```python
from build123d import *

# Parameters (mm, degrees)
F0_R     = 20
F0_R_2   = 10
F1_DEPTH = 28
F2_DEPTH = 40
F3_DEPTH = 12


with BuildPart() as f1:
    # F0 (on Front) → F1 (new body)
    with BuildSketch(Plane.XZ):
        Circle(F0_R)
        Circle(F0_R_2, mode=Mode.SUBTRACT)
    extrude(amount=F1_DEPTH)



with BuildPart() as f2:
    # F0 (on Front) → F2 (new body)
    with BuildSketch(Plane.XZ):
        Polygon((40, -40), (0, -40), (-40, -40), (-40, -70), (-20, -70), (-20, -55), (20, -55), (20, -70), (40, -70), align=None)
    extrude(amount=F2_DEPTH)


with BuildPart() as f1_1:
    add(f1.part)

    add(f2.part)  # F3 merges F2
    # F0 (on Front) → F3 (join)
    with BuildSketch(Plane.XZ):
        with BuildLine():
            ThreePointArc((0, -40), (28.2842712475, -28.2842712475), (40, 0))
            ThreePointArc((40, 0), (0, 40), (-40, 0))
            ThreePointArc((-40, 0), (-28.2842712475, -28.2842712475), (0, -40))
        make_face()
        Circle(F0_R, mode=Mode.SUBTRACT)
        with BuildLine():
            ThreePointArc((0, -40), (-28.2842712475, -28.2842712475), (-40, 0))
            Line((-40, 0), (-40, -40))
            Line((-40, -40), (0, -40))
        make_face()
        with BuildLine():
            Line((40, -40), (40, 0))
            ThreePointArc((40, 0), (28.2842712475, -28.2842712475), (0, -40))
            Line((0, -40), (40, -40))
        make_face()
    extrude(amount=F3_DEPTH)


solid = f1_1.part
```
Build history of the part. All positions in model axes, mm. A direction names the side the tool comes from. Round coordinates to 2 decimals unless told otherwise and drop trailing zeros. Loops run counter-clockwise (first coordinate to the right, second up) from the corner with the lowest first, then second, coordinate; pieces in that order, holes last. Notation, with made-up numbers: M -16,-28 L 35,-28 A23 ccw 35,-2 Z; hole C -11.75,33 d3. An arc over 180 degrees is marked long. Answer as CSV lines item,"result".
1. Cut at D-D on z = 3.5. Write the cut outline in (x, y), then the cut area to 3 significant figures.
Resolved:
outline,"M -39.85,-12 L -19.69,-12 L -19.69,-28 L -9.37,-28 L -9.37,0 L -39.85,0 Z; M 9.37,-28 L 19.69,-28 L 19.69,-12 L 39.85,-12 L 39.85,0 L 9.37,0 Z"
area,"1,060 mm²"
2. Two-plate mould, pull along Z, no slides. Class faces 5 (the flat face through (1, -26, -40)), 6 (the cylindrical face through (0.88, -5.92, 39.99)), 7 (the flat face through (30, -20, -70)): released by +Z, released by -Z, zero draft, split by the parting line, or undercut.
Resolved:
face 5,"undercut"
face 6,"released by +Z"
face 7,"released by -Z"
3. Wall check: probe 1 along Z at (x, y) = (0, -18); probe 2 along X at (y, z) = (-35.5, -56.5); probe 3 along Y at (x, z) = (-12.5, -18). Give the ranges that are in metal, low to high. Write a range as [from, to].
Resolved:
probe 1,"z = [-55, -40], [-20, -10], [10, 20]"
probe 2,"x = [-40, -20], [20, 40]"
probe 3,"y = [-12, 0]"
4. Cut at A-A on y = -21.5. Write the cut outline in (x, z).
Resolved:
outline,"M -40,-70 L -20,-70 L -20,-55 L 20,-55 L 20,-70 L 40,-70 L 40,-40 L -40,-40 Z; C 0,0 d40; hole C 0,0 d20"
5. Cut at B-B on x = 0. Write the cut outline in (y, z).
Resolved:
outline,"M -40,-55 L 0,-55 L 0,-10 L -28,-10 L -28,-20 L -12,-20 L -12,-40 L -40,-40 Z; M -28,10 L 0,10 L 0,40 L -12,40 L -12,20 L -28,20 Z"
6. 3-axis set-ups, long thin cutter, end or side, ignore diameter. For faces 1 (the flat face through (40, -15, -43)), 2 (the flat face through (-5, -28, 9)), 3 (the flat face through (0, -20, -55)), 4 (the cylindrical face through (-4.336, -19.888, -19.524)): which of +Z, -Z, +X, -X, +Y, -Y reach the whole face in a straight line?
Resolved:
face 1,"+Z, -Z, +X, +Y, -Y"
face 2,"+Z, +X, -X, -Y"
face 3,"-Z, +Y, -Y"
face 4,"-Y"
7. Flat gauge pins, fed straight in: P1, Ø3, axis at x = -13.5, y = -15.5, coming from the -Z side; P2, Ø12, axis at x = -7, z = 0.5, coming from the -Y side; P3, Ø12, axis at x = 16.5, y = -9.5, coming from the -Z side; P4, Ø1, axis at y = -14.5, z = -6, coming from the +X side. Where does each tip first touch, or does it go through?
Resolved:
P1,"stops at z = -55"
P2,"stops at y = -28"
P3,"stops at z = -70"
P4,"stops at x = 19.23"
8. Cut at C-C on y = -5. Write the cut outline in (x, z), then the cut area to 3 significant figures.
Resolved:
outline,"M -40,-70 L -20,-70 L -20,-55 L 20,-55 L 20,-70 L 40,-70 L 40,0 A40 ccw -40,0 Z; hole C 0,0 d20"
area,"7,200 mm²"
